Read the model definition and answer for the solid it produces. Units are mm, in the model's axes. A direction names the side the tool comes from. Give positions to 0.01 mm unless a question says otherwise; leave off trailing zeros. Loops run counter-clockwise (first coordinate to the right, second up) from the corner with the lowest first, then second, coordinate; pieces in that order, holes last. Notation, with made-up numbers: (-15, 17.5) -> (4, 17.5) arc R9 cw to (4, 28.5) -> close; hole circle Ø9 at (-14, -11.75). An arc over 180 degrees is marked (long way). Return JSON: item names as keys, results as strings. Group by question number.
from build123d import *

# Parameters (mm, degrees)
F1_SIZE = 0.5


with BuildPart() as f2:
    # F0 (on Front) → F2 (revolve)
    with BuildSketch(Plane.XZ):
        Polygon((-9, 9), (-9, 6), (0, 6), (0, 4), (8, 4), (8, 12.5), (5, 12.5), (5, 9), align=None)
    revolve(axis=Axis((0.124688, 0, 0), (1, 0, 0)))

    # F1
    f1_edges = [f2.edges().sort_by_distance(p)[0] for p in [
        (-9, 0, -6),
        (-9, 0, -9),
        (5, 0, -12.5),
        (8, 0, -12.5),
        (8, 0, -4),
    ]]
    chamfer(f1_edges, length=F1_SIZE)


solid = f2.part
1. Determine the mould class of faces 3 (the flat face through (0, 3.92, -1.42)), 4 (the cylindrical face through (-1.844, -8.923, -1.172)), 5 (the flat face through (5, -9, 2)) for opening direction Y: pulls with the +Y half, pulls with the -Y half, needs draft (parallel to the pull), parting line crosses it, or undercut.
2. Which of the six approach directions +Z, -Z, +X, -X, +Y, -Y give full straight-line access (tool end or side, diameter ignored) to faces 1 (the cylindrical face through (-4, 0, -6)), 2 (the cylindrical face through (3.802, 3.905, -0.867))?
3. Section A-A on y = 0 is taken. Determine the outline of the cut face in (x, z).
4. Section C-C on x = -1.5 is taken. Determine the outline of the cut face in (y, z), then the cut area to 3 significant figures.
5. Straight lines are drawn through the part: line 1 (Y direction, x = -5, z = 0); line 2 (Z direction, x = 2.5, y = 0). For each, find the intervals that lie inside material, in ascending order. Write a range as from..to.
6. Flat-ended cylindrical pins translate along their axes: pin 1 Ø2 at (x, y) = (-1.5, 5.5) entering from +Z; pin 2 Ø6 at (y, z) = (0.5, -1) entering from -X; pin 3 Ø2 at (x, z) = (1.5, -2.5) entering from +Y. Find the tip coordinate at first contact, or state that the pin passes through.
Completed:
{
 "1": {"face 3": "undercut", "face 4": "parting line crosses it", "face 5": "needs draft"},
 "2": {"face 1": "-X", "face 2": "+X, -X"},
 "3": {"outline": "(-9, -8.5) -> (-8.5, -9) -> (5, -9) -> (5, -12) -> (5.5, -12.5) -> (7.5, -12.5) -> (8, -12) -> (8, -4.5) -> (7.5, -4) -> (0, -4) -> (0, -6) -> (-8.5, -6) -> (-9, -6.5) -> close; (-9, 6.5) -> (-8.5, 6) -> (0, 6) -> (0, 4) -> (7.5, 4) -> (8, 4.5) -> (8, 12) -> (7.5, 12.5) -> (5.5, 12.5) -> (5, 12) -> (5, 9) -> (-8.5, 9) -> (-9, 8.5) -> close"},
 "4": {"outline": "circle Ø18 at (0, 0); hole circle Ø12 at (0, 0)", "area": "141 mm²"},
 "5": {"line 1": "y = -9..-6, 6..9", "line 2": "z = -9..-4, 4..9"},
 "6": {"pin 1": "stops at z = 7.79", "pin 2": "stops at x = 0", "pin 3": "stops at y = 8.87"}
}
